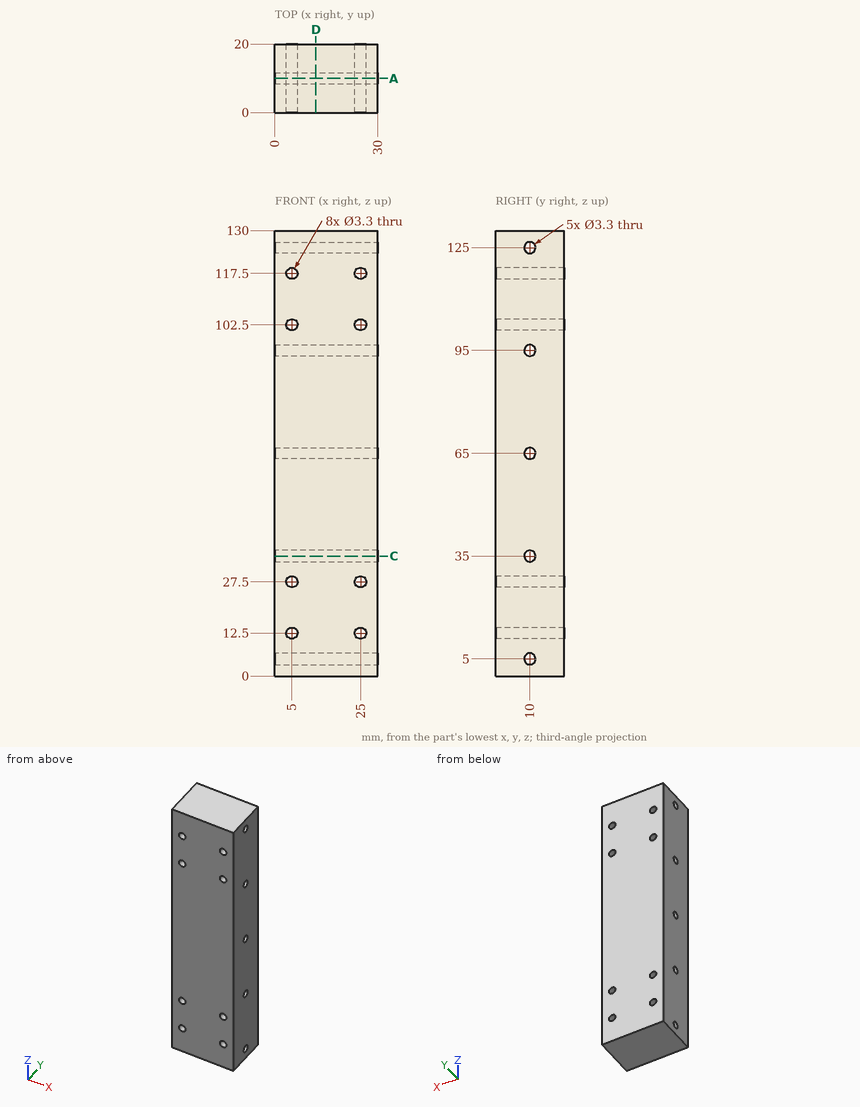
The drawing under review shows one solid part. Ordinate dimensions are in mm from its lowest x, y, z. Round coordinates to 2 decimals unless told otherwise and drop trailing zeros. Write each loop counter-clockwise with the first axis right and the second up, starting at its lowest first coordinate (ties: lowest second). Pieces come first, ordered by that corner, then holes. Notation, with made-up numbers: (84, 47.25) -> (119, 47.25) arc R25 cw to (119, 82.25) -> close; hole circle Ø8 at (83.5, 72.5). An arc over 180 degrees is marked (long way). Put each result on its own line as item: value.
Q1. Consider section A-A on y = 10. Give the number of separate pieces and of enclosed holes in the cut face, and give its area (3 significant figures).
Determined:
separate pieces: 6
enclosed holes: 8
area: 3,340 mm^2
Q2. Consider section C-C on z = 35. State the section outline as (x, y) points.
Determined:
outline: (0, 0) -> (30, 0) -> (30, 8.35) -> (0, 8.35) -> close; (0, 11.65) -> (30, 11.65) -> (30, 20) -> (0, 20) -> close
Q3. Clearance check with a flat-ended pin moving along its axis: pin 1 Ø3 at (x, z) = (25, 12.5) entering from -Y. State where the tip first meets the part, or that it passes through.
Determined:
pin 1: passes through
Q4. Consider section D-D on x = 12. State the section outline as (y, z) points, and give its area (3 significant figures).
Determined:
outline: (0, 0) -> (20, 0) -> (20, 130) -> (0, 130) -> close; hole circle Ø3.3 at (10, 5); hole circle Ø3.3 at (10, 35); hole circle Ø3.3 at (10, 65); hole circle Ø3.3 at (10, 95); hole circle Ø3.3 at (10, 125)
area: 2,560 mm^2
Q5. To check wall thickness, follow L1, parallel to X at y = 7.5, z = 27.5; L2, parallel to Z at x = 3.75, y = 12; L3, parallel to Z at x = 7.75, y = 10.75. State the ranges of each line that lie inside material, in increasing order. Write a range as [from, to].
Determined:
L1: x = [0, 3.35], [6.65, 23.35], [26.65, 30]
L2: z = [0, 11.42], [13.58, 26.42], [28.58, 101.42], [103.58, 116.42], [118.58, 130]
L3: z = [0, 3.53], [6.47, 33.53], [36.47, 63.53], [66.47, 93.53], [96.47, 123.53], [126.47, 130]
